Autodesk Inventor part; units mm, degrees
ref_plane "YZ Plane" through (0, 0, 0) normal (1, 0, 0) x (0, 1, 0)
ref_plane "XZ Plane" through (0, 0, 0) normal (0, 1, 0) x (-1, 0, 0)
ref_plane "XY Plane" through (0, 0, 0) normal (0, 0, 1) x (1, 0, 0)
sketch "Sketch1" plane through (0, 0, 0) normal (0, 0, 1) x (1, 0, 0)
  line L0 (0, 0) -> (18, 0)
  line L1 (18, 0) -> (18, 12)
  line L2 (18, 12) -> (0, 12)
  line L3 (0, 12) -> (0, 0)
  line L4 (0, 0) -> (11, 0)
  line L5 (11, 0) -> (11, 12)
  line L6 (11, 12) -> (0, 12)
  line L7 (0, 12) -> (0, 0)
  line L8 (18, 12) -> (19.5, 12)
  arc A0 (14.5, 12) -> (22.6054, 8.0813) centre (19.5, 12) ccw
  point P0 (18, 7.2303)
  dimension "d0" = 18
  dimension "d1" = 12
  dimension "d2" = 11
  dimension "d3" = 1.5
  dimension "d4" = 5
revolve "Revolution1" add sketch "Sketch1" angle 360 about axis through (0, 12, 0) along (0, -1, 0) contours L5 L2 A0 L1 L0
fillet "Fillet1" radius 0.5 2 edges at (-18, 0, 0) (-11, 0, 0)
properties part number "DriveWheelHalf"
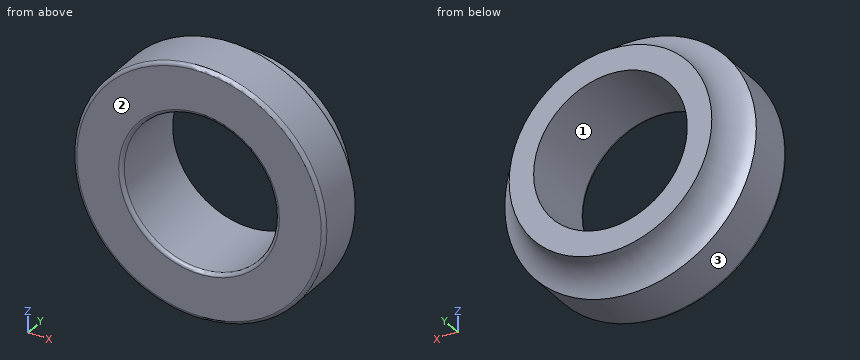
CAD build for the part. Positions are in the model's coordinates, mm. Face numbers are marked on the shaded views. Round coordinates to 2 decimals unless told otherwise and drop trailing zeros. Order: outer loops, then holes, each group sorted by start corner. A loop starts at its lowest first (then second) coordinate and runs counter-clockwise, first axis right, second up.
Q1. Slice it at A-A (x = 0). Write the cut outline in (y, z).
Q2. Wall check: L1, parallel to Z at x = 0, y = 4; L2, parallel to X at y = 3, z = -8; L3, parallel to X at y = 9, z = 4. Give the ranges that are in metal, low to high.
Q3. Slice it at C-C (y = 5.75). Write the cut outline in (x, z), and give its area (3 significant figures).
Q4. Slice it at B-B (z = 0). Write the cut outline in (x, y), and give its area (3 significant figures).
Q5. Two-plate mould, pull along Z, no slides. Class the marked faces 1, 2 and 3: pulls with the +Z half, pulls with the -Z half, needs draft (parallel to the pull), parting line crosses it, or undercut.
Q6. Drop flat-ended pins along their axis: pin 1 (2 mm diameter, centred on x = -4.5, y = 2, fed in from +Z); pin 2 (3 mm diameter, centred on x = -6.5, y = 8.5, fed in from -Z); pin 3 (3 mm diameter, centred on x = -9.5, y = 7.5, fed in from +Z). Give the stop position or say it passes through.
Results below:
1. outline: (0, -17.5) arc R0.5 ccw to (0.5, -18) - (7.23, -18) arc R5 cw to (12, -14.5) - (12, -11) - (0.5, -11) arc R0.5 ccw to (0, -11.5) - close; (0, 11.5) arc R0.5 ccw to (0.5, 11) - (12, 11) - (12, 14.5) arc R5 cw to (7.23, 18) - (0.5, 18) arc R0.5 ccw to (0, 17.5) - close
2. L1: z = -18 to -11, 11 to 18
2. L2: x = -16.12 to -7.55, 7.55 to 16.12
2. L3: x = -14.97 to -10.25, 10.25 to 14.97
3. outline: circle Ø36 at (0, 0); hole circle Ø22 at (0, 0)
3. area: 638 mm2
4. outline: (-18, 0.5) arc R0.5 ccw to (-17.5, 0) - (-11.5, 0) arc R0.5 ccw to (-11, 0.5) - (-11, 12) - (-14.5, 12) arc R5 cw to (-18, 7.23) - close; (11, 0.5) arc R0.5 ccw to (11.5, 0) - (17.5, 0) arc R0.5 ccw to (18, 0.5) - (18, 7.23) arc R5 cw to (14.5, 12) - (11, 12) - close
4. area: 143 mm2
5. face 1: undercut
5. face 2: needs draft
5. face 3: parting line crosses it
6. pin 1: stops at z = 17.66
6. pin 2: stops at z = -17.07
6. pin 3: stops at z = 16.11
